Could you check a few things on this model? Use its own coordinates, in mm. Face numbers are marked on the shaded views. A direction names the side the tool comes from. Round coordinates to 2 decimals unless told otherwise and drop trailing zeros. Loops run counter-clockwise (first coordinate to the right, second up) from the corner with the lowest first, then second, coordinate; pieces in that order, holes last.
from build123d import *

# Parameters (mm, degrees)
F1_DEPTH = 50
F4_DEPTH = 100
F5_DEPTH = 31
F6_R     = 26
F7_DEPTH = 15


with BuildPart() as f1:
    # F0 (on Front) → F1 (new body)
    with BuildSketch(Plane.XZ):
        with BuildLine():
            Line((111, 76), (0, 76))
            ThreePointArc((0, 76), (30.2492433933, 69.7207521053), (55.5, 51.9206124771))
            ThreePointArc((55.5, 51.9206124771), (80.7507566067, 69.7207521053), (111, 76))
        make_face()
        with BuildLine():
            ThreePointArc((55.5, -51.9206124771), (30.2492433933, -69.7207521053), (0, -76))
            Line((0, -76), (111, -76))
            ThreePointArc((111, -76), (80.7507566067, -69.7207521053), (55.5, -51.9206124771))
        make_face()
        with BuildLine():
            ThreePointArc((76, 0), (70.6894617323, 27.9105714739), (55.5, 51.9206124771))
            ThreePointArc((55.5, 51.9206124771), (35, 0), (55.5, -51.9206124771))
            ThreePointArc((55.5, -51.9206124771), (70.6894617323, -27.9105714739), (76, 0))
        make_face()
        with BuildLine():
            ThreePointArc((111, 76), (80.7507566067, 69.7207521053), (55.5, 51.9206124771))
            ThreePointArc((55.5, 51.9206124771), (70.6894617323, 27.9105714739), (76, 0))
            ThreePointArc((76, 0), (70.6894617323, -27.9105714739), (55.5, -51.9206124771))
            ThreePointArc((55.5, -51.9206124771), (80.7507566067, -69.7207521053), (111, -76))
            ThreePointArc((111, -76), (164.7401153702, -53.7401153702), (187, 0))
            ThreePointArc((187, 0), (164.7401153702, 53.7401153702), (111, 76))
        make_face()
        with BuildLine():
            ThreePointArc((55.5, 51.9206124771), (30.2492433933, 69.7207521053), (0, 76))
            ThreePointArc((0, 76), (-76, 0), (0, -76))
            ThreePointArc((0, -76), (30.2492433933, -69.7207521053), (55.5, -51.9206124771))
            ThreePointArc((55.5, -51.9206124771), (35, 0), (55.5, 51.9206124771))
        make_face()
    extrude(amount=F1_DEPTH)

    # F3 (on offset) + F1_face (on face) → F4 (cut)
    with BuildSketch(Plane.XZ.offset(19)):
        with BuildLine():
            ThreePointArc((55.5, 31.870833061), (32.0645184285, 55.3883260078), (0, 64))
            ThreePointArc((0, 64), (-64, 0), (0, -64))
            ThreePointArc((0, -64), (32.0645184285, -55.3883260078), (55.5, -31.870833061))
            ThreePointArc((55.5, -31.870833061), (47, 0), (55.5, 31.870833061))
        make_face()
        with BuildLine():
            Line((111, 64), (0, 64))
            ThreePointArc((0, 64), (32.0645184285, 55.3883260078), (55.5, 31.870833061))
            ThreePointArc((55.5, 31.870833061), (78.9354815715, 55.3883260078), (111, 64))
        make_face()
        with BuildLine():
            ThreePointArc((55.5, -31.870833061), (32.0645184285, -55.3883260078), (0, -64))
            Line((0, -64), (111, -64))
            ThreePointArc((111, -64), (78.9354815715, -55.3883260078), (55.5, -31.870833061))
        make_face()
        with BuildLine():
            ThreePointArc((111, 64), (78.9354815715, 55.3883260078), (55.5, 31.870833061))
            ThreePointArc((55.5, 31.870833061), (61.838499335, 16.4924225025), (64, 0))
            ThreePointArc((64, 0), (61.838499335, -16.4924225025), (55.5, -31.870833061))
            ThreePointArc((55.5, -31.870833061), (78.9354815715, -55.3883260078), (111, -64))
            ThreePointArc((111, -64), (156.2548339959, -45.2548339959), (175, 0))
            ThreePointArc((175, 0), (156.2548339959, 45.2548339959), (111, 64))
        make_face()
    with BuildSketch(Plane(origin=(55.5, -50, 0), x_dir=(1, 0, 0), z_dir=(0, -1, 0))):
        with BuildLine():
            Line((55.5, 76), (-55.5, 76))
            ThreePointArc((-55.5, 76), (-131.5, 0), (-55.5, -76))
            Line((-55.5, -76), (55.5, -76))
            ThreePointArc((55.5, -76), (131.5, 0), (55.5, 76))
        make_face()
    extrude(amount=F4_DEPTH, mode=Mode.SUBTRACT)

    # F5 (cut, through all): a face of the model
    f5_faces = [f1.faces().sort_by_distance(p)[0] for p in [
        (55.5, -50, 0),
    ]]
    extrude(f5_faces, amount=-F5_DEPTH, mode=Mode.SUBTRACT)

    # F6 (on offset) → F7 (cut)
    with BuildSketch(Plane.XZ.offset(19)):
        Circle(F6_R)
    extrude(amount=-F7_DEPTH, mode=Mode.SUBTRACT)

    # F9 (on offset) → F10 (revolve, cut)
    with BuildSketch(Plane.YZ.offset(111)):
        Polygon((-19, 0), (0, 0), (0, 11), (-2, 11), (-2, 18.6120123814), (-7, 18.6120123814), (-7, 23.182326171), (-19, 23.182326171), align=None)
    revolve(axis=Axis((111, -26.2971315533, 0), (0, -1, 0)), mode=Mode.SUBTRACT)


solid = f1.part
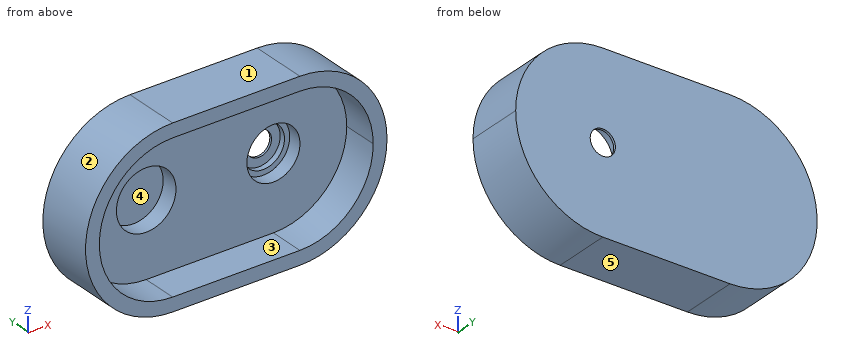
Item 1: If I drill on line 1 along Z through (x, y) = (111, -3); line 2 along X through (y, z) = (-0.9, 0); line 3 along Z through (x, y) = (10, -45.5), over which ranges is the centre line in solid material (lowest first)?
Results list:
line 1: z = -76 to -18.61, 18.61 to 76
line 2: x = -76 to 100, 122 to 187
line 3: z = -76 to -64, 64 to 76
Item 2: We'd pull the mould along X, two halves only. Please class the marked faces 1, 2 and 3: released by +X, released by -X, zero draft, split by the parting line, or undercut.
Results list:
face 1: zero draft
face 2: released by -X
face 3: undercut
Item 3: If we section it at A-A, the plane y = -37.5: Please give me the cut outline in (x, z), then the cut area to 3 significant figures.
Results list:
outline: (0, -76) - (111, -76) arc R76 ccw to (111, 76) - (0, 76) arc R76 ccw to start; hole (0, -64) - (111, -64) arc R64 ccw to (111, 64) - (0, 64) arc R64 ccw to start
area: 7,940 mm2
Item 4: Will these pins go through, and if not, where does the flat tip stop? pin 1 (10 mm diameter, centred on y = -8, z = -42, fed in from -X); pin 2 (10 mm diameter, centred on y = -31.5, z = -15, fed in from +X); pin 3 (2 mm diameter, centred on y = -34, z = 43.5, fed in from +X); pin 4 (2 mm diameter, centred on x = 8.5, z = -45.5, fed in from +Y).
Results list:
pin 1: stops at x = -66.39
pin 2: stops at x = 186.34
pin 3: stops at x = 174.01
pin 4: stops at y = 0
Item 5: If we section it at C-C, the plane z = 59: Please give me the cut outline in (x, y).
Results list:
outline: (-47.91, -50) - (-24.8, -50) - (-24.8, -19) - (135.8, -19) - (135.8, -50) - (158.91, -50) - (158.91, 0) - (-47.91, 0) - close
Item 6: For the marked faces 4 and 5, which set-ups out of +Z, -Z, +X, -X, +Y, -Y let a thin tool reach every point of the face, with its end or its side?
Results list:
face 4: -Y
face 5: -Z, +X, -X, +Y, -Y
Item 7: If we section it at D-D, the plane x = 159: Please give me the cut outline in (y, z).
Results list:
outline: (-50, -58.92) - (0, -58.92) - (0, 58.92) - (-50, 58.92) - (-50, 42.33) - (-19, 42.33) - (-19, -42.33) - (-50, -42.33) - close
Item 8: If we section it at B-B, the plane y = -16: Please give me the cut outline in (x, z).
Results list:
outline: (0, -76) - (111, -76) arc R76 ccw to (111, 76) - (0, 76) arc R76 ccw to start; hole circle Ø52 at (0, 0); hole circle Ø46.36 at (111, 0)
